The listing builds one solid part. Answer for the finished solid, in the listing's coordinates (mm). Face numbers are marked on the shaded views. A direction names the side the tool comes from. Coordinates: 2 decimals unless noted, no trailing zeros. Order: outer loops, then holes, each group sorted by start corner. A loop starts at its lowest first (then second) coordinate and runs counter-clockwise, first axis right, second up. Notation, with made-up numbers: (73, 28) -> (92, 28) arc R25 cw to (92, 47) -> close; hole circle Ø9 at (53, 21.5). An arc over 180 degrees is marked (long way). Write item = value, one per line.
from build123d import *

# Parameters (mm, degrees)
Y_KSEKLIK_EKSTR_ZYON1_DEPTH       = 3
Y_KSEKLIK_EKSTR_ZYON1_DEPTH_BACK  = 3
IZIM1_R                           = 1.25
IZIM2_W                           = 2
IZIM2_H                           = 2
Y_KSEKLIK_EKSTR_ZYON2_DEPTH       = 1.5
Y_KSEKLIK_EKSTR_ZYON6_DEPTH       = 3.1
Y_KSEKLIK_EKSTR_ZYON6_DEPTH_BACK  = 3.1
KES_EKSTR_ZYON1_DEPTH             = 6
KES_EKSTR_ZYON1_DEPTH_BACK        = 0.5
IZIM5_W                           = 5
IZIM5_H                           = 3.50112481
KES_EKSTR_ZYON2_DEPTH             = 5.25
Y_KSEKLIK_EKSTR_ZYON7_DEPTH       = 1.25
Y_KSEKLIK_EKSTR_ZYON7_DEPTH_BACK  = 1.25
IZIM6_R                           = 2
Y_KSEKLIK_EKSTR_ZYON8_DEPTH       = 2.2
Y_KSEKLIK_EKSTR_ZYON8_DEPTH_BACK  = 2.2
IZIM7_R                           = 1
Y_KSEKLIK_EKSTR_ZYON9_DEPTH       = 0.25
Y_KSEKLIK_EKSTR_ZYON9_DEPTH_BACK  = 0.25
Y_KSEKLIK_EKSTR_ZYON10_DEPTH      = 0.25
Y_KSEKLIK_EKSTR_ZYON10_DEPTH_BACK = 0.25
Y_KSEKLIK_EKSTR_ZYON11_DEPTH      = 0.25
Y_KSEKLIK_EKSTR_ZYON11_DEPTH_BACK = 0.25
KES_EKSTR_ZYON3_REACH             = 25.675
IZIM11_R                          = 0.75
Y_KSEKLIK_EKSTR_ZYON13_DEPTH      = 3.2
Y_KSEKLIK_EKSTR_ZYON13_DEPTH_BACK = 3.2
IZIM13_R                          = 0.5


with BuildPart() as part:
    # izim1 → Y_kseklik-Ekstr_zyon1 (new, two sides: drawn at the far end of the back side and taken through both)
    with BuildSketch(Plane(origin=(0, 0, 0), x_dir=(1, 0, 0), z_dir=(0, 1, 0)).offset(-Y_KSEKLIK_EKSTR_ZYON1_DEPTH_BACK)):
        with BuildLine():
            Line((0.207106781, 5.5), (9.5, 5.5))
            ThreePointArc((9.5, 5.5), (9.853553391, 5.353553391), (10, 5))
            Line((10, 5), (10, -5.5))
            Line((10, -5.5), (-10, -5.5))
            Line((-10, -5.5), (-10, 4))
            ThreePointArc((-10, 4), (-9.853553391, 4.353553391), (-9.5, 4.5))
            Line((-9.5, 4.5), (-1.207106781, 4.5))
            ThreePointArc((-1.207106781, 4.5), (-1.015765065, 4.538060234), (-0.853553391, 4.646446609))
            Line((-0.853553391, 4.646446609), (-0.146446609, 5.353553391))
            ThreePointArc((-0.146446609, 5.353553391), (0.015765065, 5.461939766), (0.207106781, 5.5))
        make_face()
        with Locations(Location((-4.75, -4.125, 0), (0, 0, 270))):
            Circle(IZIM1_R, mode=Mode.SUBTRACT)
        with Locations(Location((4.75, -4.125, 0), (0, 0, 90))):
            Circle(IZIM1_R, mode=Mode.SUBTRACT)
    extrude(amount=Y_KSEKLIK_EKSTR_ZYON1_DEPTH + Y_KSEKLIK_EKSTR_ZYON1_DEPTH_BACK)

    # izim2 → Y_kseklik-Ekstr_zyon2 (add)
    with BuildSketch(Plane(origin=(0, 0, -5.5), x_dir=(-1, 0, 0), z_dir=(0, 0, -1))):
        with Locations((-1.853553391, 0)):
            Rectangle(IZIM2_W, IZIM2_H)
    extrude(amount=Y_KSEKLIK_EKSTR_ZYON2_DEPTH)

    # izim3 → Y_kseklik-Ekstr_zyon6 (add, two sides: drawn at the far end of the back side and taken through both)
    with BuildSketch(Plane(origin=(0, 0, 0), x_dir=(1, 0, 0), z_dir=(0, 1, 0)).offset(-Y_KSEKLIK_EKSTR_ZYON6_DEPTH_BACK)):
        with BuildLine():
            Line((9.5, 5.5), (8.993860128, 3.307667354))
            ThreePointArc((8.993860128, 3.307667354), (8.438296627, 2.528796052), (7.494708729, 2.370893591))
            Line((7.494708729, 2.370893591), (7.007523696, 2.483369118))
            ThreePointArc((7.007523696, 2.483369118), (6.228652394, 3.038932619), (6.070749933, 3.982520517))
            Line((6.070749933, 3.982520517), (6.576889806, 6.174853163))
            Line((6.576889806, 6.174853163), (-8.038661166, 9.549118978))
            Line((-8.038661166, 9.549118978), (-7.116361843, 13.544036244))
            ThreePointArc((-7.116361843, 13.544036244), (-6.494130723, 14.416372102), (-5.437312277, 14.593222858))
            Line((-5.437312277, 14.593222858), (-4.755253231, 14.43575712))
            ThreePointArc((-4.755253231, 14.43575712), (-3.882917373, 13.813526), (-3.706066617, 12.756707554))
            Line((-3.706066617, 12.756707554), (-4.583375729, 8.956664301))
            Line((-4.583375729, 8.956664301), (9.544990211, 5.694874013))
            Line((9.544990211, 5.694874013), (9.5, 5.5))
        make_face()
    extrude(amount=Y_KSEKLIK_EKSTR_ZYON6_DEPTH + Y_KSEKLIK_EKSTR_ZYON6_DEPTH_BACK)

    # izim4 → Kes-Ekstr_zyon1 (cut, two sides: drawn at the far end of the back side and taken through both)
    with BuildSketch(Plane(origin=(1.731239145, 0, -7.498820588), x_dir=(-0.9743700647852337, 0, -0.2249510543438719), z_dir=(0.22495105434387186, 0, -0.9743700647852336)).offset(-KES_EKSTR_ZYON1_DEPTH_BACK)):
        Polygon((-5.019284817, 2.500562405), (-4.519284817, 2.000562405), (10.019957698, 2.000562405), (10.019957698, 3.1), (-5.019284817, 3.1), align=None)
        Polygon((-4.519284817, -2.000562405), (10.019957698, -2.000562405), (10.019957698, -3.1), (-5.019284817, -3.1), (-5.019284817, -2.500562405), align=None)
    extrude(amount=KES_EKSTR_ZYON1_DEPTH + KES_EKSTR_ZYON1_DEPTH_BACK, mode=Mode.SUBTRACT)

    # izim5 → Kes-Ekstr_zyon2 (cut)
    with BuildSketch(Plane(origin=(2.923479733, 0, -12.662981931), x_dir=(-0.9743700647852332, 0, -0.2249510543438736), z_dir=(0.2249510543438736, 0, -0.9743700647852332))):
        with Locations((8.230715183, 0)):
            Rectangle(IZIM5_W, IZIM5_H)
    extrude(amount=-KES_EKSTR_ZYON2_DEPTH, mode=Mode.SUBTRACT)



with BuildPart() as body_2:
    # izim6 → Y_kseklik-Ekstr_zyon7 (new, two sides: drawn at the far end of the back side and taken through both)
    with BuildSketch(Plane(origin=(0, 0.000562405, 0), x_dir=(1, 0, 0), z_dir=(0, 1, 0)).offset(-Y_KSEKLIK_EKSTR_ZYON7_DEPTH_BACK)):
        with Locations(Location((-5.431324974, 13.063262696, 0), (0, 0, 270))):
            Circle(IZIM6_R)
    extrude(amount=Y_KSEKLIK_EKSTR_ZYON7_DEPTH + Y_KSEKLIK_EKSTR_ZYON7_DEPTH_BACK)


with BuildPart() as part_1:
    add(part.part)

    add(body_2.part)  # Y_kseklik-Ekstr_zyon8 merges body 2
    # izim7 → Y_kseklik-Ekstr_zyon8 (add, two sides: drawn at the far end of the back side and taken through both)
    with BuildSketch(Plane(origin=(0, 0.000562405, 0), x_dir=(1, 0, 0), z_dir=(0, 1, 0)).offset(-Y_KSEKLIK_EKSTR_ZYON8_DEPTH_BACK)):
        with Locations(Location((-5.431324974, 13.063262696, 0), (0, 0, 270))):
            Circle(IZIM7_R)
    extrude(amount=Y_KSEKLIK_EKSTR_ZYON8_DEPTH + Y_KSEKLIK_EKSTR_ZYON8_DEPTH_BACK)

    # izim8 → Y_kseklik-Ekstr_zyon9 (add, two sides: drawn at the far end of the back side and taken through both)
    with BuildSketch(Plane.ZY.offset(8.25).offset(-Y_KSEKLIK_EKSTR_ZYON9_DEPTH_BACK)):
        with BuildLine():
            Line((5.5, 1.5), (5.5, -1.5))
            Line((5.5, -1.5), (9.25, -1.5))
            ThreePointArc((9.25, -1.5), (9.426776695, -1.426776695), (9.5, -1.25))
            Line((9.5, -1.25), (9.5, 1.25))
            ThreePointArc((9.5, 1.25), (9.426776695, 1.426776695), (9.25, 1.5))
            Line((9.25, 1.5), (5.5, 1.5))
        make_face()
    extrude(amount=Y_KSEKLIK_EKSTR_ZYON9_DEPTH + Y_KSEKLIK_EKSTR_ZYON9_DEPTH_BACK)

    # izim9 → Y_kseklik-Ekstr_zyon10 (add, two sides: drawn at the far end of the back side and taken through both)
    with BuildSketch(Plane(origin=(7.75, 0, 0), x_dir=(0, 0, -1), z_dir=(1, 0, 0)).offset(-Y_KSEKLIK_EKSTR_ZYON10_DEPTH_BACK)):
        with BuildLine():
            Line((-5.5, 1.5), (-9.264217475, 1.5))
            ThreePointArc((-9.264217475, 1.5), (-9.44099417, 1.426776695), (-9.514217475, 1.25))
            Line((-9.514217475, 1.25), (-9.514217475, -1.25))
            ThreePointArc((-9.514217475, -1.25), (-9.44099417, -1.426776695), (-9.264217475, -1.5))
            Line((-9.264217475, -1.5), (-5.5, -1.5))
            Line((-5.5, -1.5), (-5.5, 1.5))
        make_face()
    extrude(amount=Y_KSEKLIK_EKSTR_ZYON10_DEPTH + Y_KSEKLIK_EKSTR_ZYON10_DEPTH_BACK)

    # izim10 → Y_kseklik-Ekstr_zyon11 (add, two sides: drawn at the far end of the back side and taken through both)
    with BuildSketch(Plane(origin=(-1, 0, 0), x_dir=(0, 0, -1), z_dir=(1, 0, 0)).offset(-Y_KSEKLIK_EKSTR_ZYON11_DEPTH_BACK)):
        with BuildLine():
            Line((-5.5, 1.5), (-9.25, 1.5))
            ThreePointArc((-9.25, 1.5), (-9.426776695, 1.426776695), (-9.5, 1.25))
            Line((-9.5, 1.25), (-9.5, -1.25))
            ThreePointArc((-9.5, -1.25), (-9.426776695, -1.426776695), (-9.25, -1.5))
            Line((-9.25, -1.5), (-5.5, -1.5))
            Line((-5.5, -1.5), (-5.5, 1.5))
        make_face()
    extrude(amount=Y_KSEKLIK_EKSTR_ZYON11_DEPTH + Y_KSEKLIK_EKSTR_ZYON11_DEPTH_BACK)

    # Kes-Ekstr_zyon3: up to this face of the body (flat: up to its plane)
    kes_ekstr_zyon3_end = Plane(part_1.part.faces().sort_by_distance((-10, 0, 0.75))[0])
    # izim11 → Kes-Ekstr_zyon3 (cut, up to the picked face)
    with BuildSketch(Plane(origin=(8, 0, 0), x_dir=(0, 0, -1), z_dir=(1, 0, 0)), mode=Mode.PRIVATE) as kes_ekstr_zyon3_sk1:
        with Locations(Location((-7.764217475, 0, 0), (0, 0, 180))):
            Circle(IZIM11_R)
    kes_ekstr_zyon3_tool1 = split(extrude(kes_ekstr_zyon3_sk1.sketch, amount=-KES_EKSTR_ZYON3_REACH, mode=Mode.PRIVATE), bisect_by=kes_ekstr_zyon3_end, keep=Keep.BOTH, mode=Mode.PRIVATE)
    add(kes_ekstr_zyon3_tool1.solids().sort_by(Axis((8, 0, 7.764217), (-1, 0, 0)))[0], mode=Mode.SUBTRACT)

    # izim13 → Y_kseklik-Ekstr_zyon13 (add, two sides: drawn at the far end of the back side and taken through both)
    with BuildSketch(Plane(origin=(0, 0, 0), x_dir=(1, 0, 0), z_dir=(0, 1, 0)).offset(-Y_KSEKLIK_EKSTR_ZYON13_DEPTH_BACK)):
        with Locations(Location((7.588542794, 3.888686452, 0), (0, 0, 270))):
            Circle(IZIM13_R)
    extrude(amount=Y_KSEKLIK_EKSTR_ZYON13_DEPTH + Y_KSEKLIK_EKSTR_ZYON13_DEPTH_BACK)


solid = part_1.part
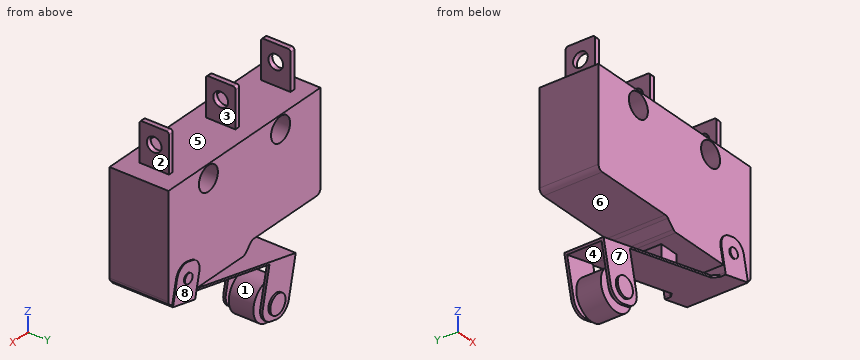
Q1. The mould has two halves that part along Z. Classify the marked faces 5, 6, 7 and 8: released by +Z, released by -Z, zero draft, split by the parting line, or undercut.
The answers:
face_5 = released by +Z
face_6 = undercut
face_7 = undercut
face_8 = zero draft
Q2. Section C-C, the plane z = 7.75 is taken. Give the vertices of the cut face in (x, y).
The answers:
outline = (-8.5, -1.5) -> (-8, -1.5) -> (-8, -0.75) -> (-8.5, -0.75) -> close; (-8.5, 0.75) -> (-8, 0.75) -> (-8, 1.5) -> (-8.5, 1.5) -> close; (-1.25, -1.5) -> (-0.75, -1.5) -> (-0.75, -0.75) -> (-1.25, -0.75) -> close; (-1.25, 0.75) -> (-0.75, 0.75) -> (-0.75, 1.5) -> (-1.25, 1.5) -> close; (7.5, -1.5) -> (8, -1.5) -> (8, -0.75) -> (7.5, -0.75) -> close; (7.5, 0.75) -> (8, 0.75) -> (8, 1.5) -> (7.5, 1.5) -> close
Q3. Section D-D, the plane z = 1 is taken. Give the vertices of the cut face in (x, y), plus the area to 3 significant figures.
The answers:
outline = (-10, -3) -> (10, -3) -> (10, 3) -> (-10, 3) -> close
area = 120 mm2
Q4. Section A-A, the plane x = -2.5 is taken. Give the vertices of the cut face in (y, z), plus the area to 3 significant figures.
The answers:
outline = (-3, -4.5) -> (3, -4.5) -> (3, 5.5) -> (-3, 5.5) -> close; (-2, -8.48) -> (2, -8.48) -> (2, -8.27) -> (-2, -8.27) -> close
area = 60.8 mm2
Q5. A tool of negligible diameter and unlimited length cuts with its end or side. For the marked faces 1, 2, 3 and 4, from which of +Z, -Z, +X, -X, +Y, -Y can it reach the whole face along a straight path? Write none if from no direction.
The answers:
face_1 = none
face_2 = +Z, +X, +Y, -Y
face_3 = +Z, +Y, -Y
face_4 = +X
Q6. Each of these flat-tipped pins is pushed along its axis until it touches: pin 1 Ø1.2 at (x, z) = (2.5, -6) entering from +Y; pin 2 Ø1 at (x, z) = (-5, -13.5) entering from -Y; pin 3 Ø0.6 at (x, y) = (1.5, 0) entering from -Z. Where does it stop, or does it pass through?
The answers:
pin_1 = 3
pin_2 = -2.2
pin_3 = -7.62
Q7. Find the intervals of material crossed by line 1 along Z through (x, y) = (4.25, -0.25); line 2 along Z through (x, y) = (4, 1.5) (3 decimals); line 3 along Y through (x, z) = (-6, -12.5), in increasing order.
The answers:
line_1 = -6.92 to -6.71, -5.5 to 2.98, 5.27 to 5.5
line_2 = -6.975 to -6.77, -5.5 to 3.125, 5.125 to 5.5
line_3 = -2.2 to 2.2
Q8. Section B-B, the plane x = 4.75 is taken. Give the vertices of the cut face in (y, z) (3 decimals).
The answers:
outline = (-3, -5.5) -> (3, -5.5) -> (3, 2.875) -> (-3, 2.875) -> close; (-3, 5.375) -> (3, 5.375) -> (3, 5.5) -> (-3, 5.5) -> close; (-2.001, -6.802) -> (2.001, -6.802) -> (2.001, -6.597) -> (-2.001, -6.597) -> close
